```python
from build123d import *

# Parameters (mm, degrees)
SKETCH1_W           = 92.3798
SKETCH1_H           = 35.56
SKETCH1_R           = 7.62
BOSS_EXTRUDE1_DEPTH = 10.16
FILLET1_R           = 1.27
FILLET2_R           = 1.27
FILLET3_R           = 17.78
FILLET4_R           = 10.16
FILLET5_R           = 12.7
FILLET6_R           = 12.7


with BuildPart() as part:
    # Sketch1 → Boss-Extrude1 (new body)
    with BuildSketch(Plane.XY):
        with Locations((46.1899, 17.78)):
            Rectangle(SKETCH1_W, SKETCH1_H)
        with Locations((25.4, 17.78)):
            Circle(SKETCH1_R, mode=Mode.SUBTRACT)
    extrude(amount=BOSS_EXTRUDE1_DEPTH)

    # Fillet1
    fillet1_edges = [part.edges().sort_by_distance(p)[0] for p in [
        (46.1899, 35.56, 10.16),
        (0, 17.78, 10.16),
        (46.1899, 0, 10.16),
        (92.3798, 17.78, 10.16),
    ]]
    fillet(fillet1_edges, radius=FILLET1_R)

    # Fillet2
    fillet2_edges = [part.edges().sort_by_distance(p)[0] for p in [
        (0, 17.78, 0),
        (46.1899, 35.56, 0),
        (92.3798, 17.78, 0),
        (46.1899, 0, 0),
    ]]
    fillet(fillet2_edges, radius=FILLET2_R)

    # Fillet3
    # the kernel refuses this fillet: 17.78 mm, written as the material it takes off along each edge
    with BuildSketch(Plane(origin=(74.5998, 17.78, 10.16), x_dir=(0, -1, 0), z_dir=(-1, 0, 0))) as fillet3_piece_1:
        with BuildLine():
            CenterArc((16.51, -1.27), 1.27, 0, 90)
            Line((17.78, -1.27), (17.78, 0))
            Line((17.78, 0), (16.51, 0))
        make_face()
    revolve(axis=Axis((74.5998, 17.78, 10.16), (0, 0, 1)), revolution_arc=90, mode=Mode.SUBTRACT)
    with BuildSketch(Plane(origin=(74.5998, 17.78, 0), x_dir=(1, 0, 0), z_dir=(0, 1, 0))) as fillet3_piece_2:
        with BuildLine():
            CenterArc((16.51, -1.27), 1.27, 0, 90)
            Line((17.78, -1.27), (17.78, 0))
            Line((17.78, 0), (16.51, 0))
        make_face()
    revolve(axis=Axis((74.5998, 17.78, 0), (0, 0, -1)), revolution_arc=90, mode=Mode.SUBTRACT)
    with BuildSketch(Plane(origin=(92.3798, 0, 0), x_dir=(-1, 0, 0), z_dir=(0, 0, 1))) as fillet3_piece_3:
        with BuildLine():
            CenterArc((FILLET3_R, -FILLET3_R), FILLET3_R, 90, 90)
            Line((0, -FILLET3_R), (0, 0))
            Line((0, 0), (FILLET3_R, 0))
        make_face()
    extrude(amount=10.16, mode=Mode.SUBTRACT)

    # Fillet4
    # the kernel refuses this fillet: 10.16 mm, written as the material it takes off along each edge
    with BuildSketch(Plane(origin=(82.2198, 25.4, 10.16), x_dir=(1, 0, 0), z_dir=(0, -1, 0))) as fillet4_piece_1:
        with BuildLine():
            CenterArc((8.89, -1.27), 1.27, 0, 90)
            Line((10.16, -1.27), (10.16, 0))
            Line((10.16, 0), (8.89, 0))
        make_face()
    revolve(axis=Axis((82.2198, 25.4, 10.16), (0, 0, 1)), revolution_arc=90, mode=Mode.SUBTRACT)
    with BuildSketch(Plane(origin=(82.2198, 25.4, 0), x_dir=(0, 1, 0), z_dir=(-1, 0, 0))) as fillet4_piece_2:
        with BuildLine():
            CenterArc((8.89, -1.27), 1.27, 0, 90)
            Line((10.16, -1.27), (10.16, 0))
            Line((10.16, 0), (8.89, 0))
        make_face()
    revolve(axis=Axis((82.2198, 25.4, 0), (0, 0, -1)), revolution_arc=90, mode=Mode.SUBTRACT)
    with BuildSketch(Plane(origin=(92.3798, 35.56, 0), x_dir=(-1, 0, 0), z_dir=(0, 0, 1))) as fillet4_piece_3:
        with BuildLine():
            CenterArc((FILLET4_R, FILLET4_R), FILLET4_R, 180, 90)
            Line((0, FILLET4_R), (0, 0))
            Line((0, 0), (FILLET4_R, 0))
        make_face()
    extrude(amount=10.16, mode=Mode.SUBTRACT)

    # Fillet5
    # the kernel refuses this fillet: 12.7 mm, written as the material it takes off along each edge
    with BuildSketch(Plane(origin=(12.7, 22.86, 10.16), x_dir=(0, 1, 0), z_dir=(1, 0, 0))) as fillet5_piece_1:
        with BuildLine():
            CenterArc((11.43, -1.27), 1.27, 0, 90)
            Line((12.7, -1.27), (12.7, 0))
            Line((12.7, 0), (11.43, 0))
        make_face()
    revolve(axis=Axis((12.7, 22.86, 10.16), (0, 0, 1)), revolution_arc=90, mode=Mode.SUBTRACT)
    with BuildSketch(Plane(origin=(12.7, 22.86, 0), x_dir=(-1, 0, 0), z_dir=(0, -1, 0))) as fillet5_piece_2:
        with BuildLine():
            CenterArc((11.43, -1.27), 1.27, 0, 90)
            Line((12.7, -1.27), (12.7, 0))
            Line((12.7, 0), (11.43, 0))
        make_face()
    revolve(axis=Axis((12.7, 22.86, 0), (0, 0, -1)), revolution_arc=90, mode=Mode.SUBTRACT)
    with BuildSketch(Plane(origin=(0, 35.56, 0), x_dir=(0, -1, 0), z_dir=(0, 0, 1))) as fillet5_piece_3:
        with BuildLine():
            CenterArc((FILLET5_R, FILLET5_R), FILLET5_R, 180, 90)
            Line((0, FILLET5_R), (0, 0))
            Line((0, 0), (FILLET5_R, 0))
        make_face()
    extrude(amount=10.16, mode=Mode.SUBTRACT)

    # Fillet6
    # the kernel refuses this fillet: 12.7 mm, written as the material it takes off along each edge
    with BuildSketch(Plane(origin=(12.7, 12.7, 10.16), x_dir=(-1, 0, 0), z_dir=(0, 1, 0))) as fillet6_piece_1:
        with BuildLine():
            CenterArc((11.43, -1.27), 1.27, 0, 90)
            Line((12.7, -1.27), (12.7, 0))
            Line((12.7, 0), (11.43, 0))
        make_face()
    revolve(axis=Axis((12.7, 12.7, 10.16), (0, 0, 1)), revolution_arc=90, mode=Mode.SUBTRACT)
    with BuildSketch(Plane(origin=(12.7, 12.7, 0), x_dir=(0, -1, 0), z_dir=(1, 0, 0))) as fillet6_piece_2:
        with BuildLine():
            CenterArc((11.43, -1.27), 1.27, 0, 90)
            Line((12.7, -1.27), (12.7, 0))
            Line((12.7, 0), (11.43, 0))
        make_face()
    revolve(axis=Axis((12.7, 12.7, 0), (0, 0, -1)), revolution_arc=90, mode=Mode.SUBTRACT)
    with BuildSketch(Plane(origin=(0, 0, 0), x_dir=(0, 1, 0), z_dir=(0, 0, 1))) as fillet6_piece_3:
        with BuildLine():
            CenterArc((FILLET6_R, -FILLET6_R), FILLET6_R, 90, 90)
            Line((0, -FILLET6_R), (0, 0))
            Line((0, 0), (FILLET6_R, 0))
        make_face()
    extrude(amount=10.16, mode=Mode.SUBTRACT)


solid = part.part
```
Part model, mm, in its own coordinate system. Coordinates: 2 decimals unless noted, no trailing zeros. Loops run counter-clockwise (first coordinate to the right, second up) from the corner with the lowest first, then second, coordinate; pieces in that order, holes last. Notation, with made-up numbers: (82.5, -15) - (118.5, -15) arc R16 ccw to (118.5, -8) - close; hole circle Ø9 at (34, 20). An arc over 180 degrees is marked (long way). Write item = value, one per line. Start each with the question number.
Item 1: Wall check: L1, parallel to X at y = 17.5, z = 8.5; L2, parallel to Y at x = 25.4, z = 2.5; L3, parallel to X at y = 15.5, z = 4.75. Give the ranges that are in metal, low to high. Write a range as from..to.
Item 2: Cut at A-A, the plane z = 4.5. Give the cut face in (x, y).
Item 3: Cut at C-C, the plane y = 19. Give the cut face in (x, z).
Item 4: Mould opens along X. For faces 1 (the flat face through (92.38, 22, 5)), 2 (the cylindrical face through (17.787, 18.115, 5.009)), 3 (the cylindrical face through (3.82, 31.94, 5.03)) say: released by +X, released by -X, zero draft, split by the parting line, or undercut.
Item 5: Cut at B-B, the plane x = 25.4. Give the cut face in (y, z), and give its area (3 significant figures).
Item 6: Flat gauge pins, fed straight in: pin 1 Ø1 at (x, z) = (79, 1.5) entering from -Y; pin 2 Ø5 at (y, z) = (5, 6) entering from -X. Where does each tip first touch, or does it go through?
The answers:
q1.L1 = 0..17.79, 33.01..92.38
q1.L2 = 0..10.16, 25.4..35.56
q1.L3 = 0..18.13, 32.67..92.23
q2.outline = (0, 12.7) arc R12.7 ccw to (12.7, 0) - (74.6, 0) arc R17.78 ccw to (92.38, 17.78) - (92.38, 25.4) arc R10.16 ccw to (82.22, 35.56) - (12.7, 35.56) arc R12.7 ccw to (0, 22.86) - close; hole circle Ø15.24 at (25.4, 17.78)
q3.outline = (0, 1.27) arc R1.27 ccw to (1.27, 0) - (17.88, 0) - (17.88, 10.16) - (1.27, 10.16) arc R1.27 ccw to (0, 8.89) - close; (32.92, 0) - (91.11, 0) arc R1.27 ccw to (92.38, 1.27) - (92.38, 8.89) arc R1.27 ccw to (91.11, 10.16) - (32.92, 10.16) - close
q4.face_1 = released by +X
q4.face_2 = undercut
q4.face_3 = released by -X
q5.outline = (0, 1.27) arc R1.27 ccw to (1.27, 0) - (10.16, 0) - (10.16, 10.16) - (1.27, 10.16) arc R1.27 ccw to (0, 8.89) - close; (25.4, 0) - (34.29, 0) arc R1.27 ccw to (35.56, 1.27) - (35.56, 8.89) arc R1.27 ccw to (34.29, 10.16) - (25.4, 10.16) - close
q5.area = 205 mm2
q6.pin_1 = 0.43
q6.pin_2 = 1.11
